from build123d import *

# Parameters (mm, degrees)
SKETCH2_W           = 154.686
SKETCH2_H           = 228.6
BOSS_EXTRUDE1_DEPTH = 6.35
SKETCH1_R           = 2.2225
CUT_EXTRUDE1_DEPTH  = 6.35
SKETCH3_W           = 15.24
SKETCH3_H           = 50.8
CUT_EXTRUDE2_DEPTH  = 6.35
SKETCH8_R           = 2.54
CUT_EXTRUDE3_DEPTH  = 17.78
SKETCH9_R           = 1.5875
CUT_EXTRUDE4_DEPTH  = 17.78
SKETCH10_R          = 1.5875
CUT_EXTRUDE5_DEPTH  = 10.16
SKETCH12_W          = 3.048
SKETCH12_H          = 18.542
CUT_EXTRUDE7_DEPTH  = 8.255


with BuildPart() as part:
    # Sketch2 → Boss-Extrude1 (new body)
    with BuildSketch(Plane(origin=(0, 0, 0), x_dir=(1, 0, 0), z_dir=(0, 1, 0))):
        with Locations((26.543, 26.944051327)):
            Rectangle(SKETCH2_W, SKETCH2_H)
    extrude(amount=BOSS_EXTRUDE1_DEPTH)

    # Sketch1 → Cut-Extrude1 (cut)
    with BuildSketch(Plane(origin=(0, 0, 0), x_dir=(1, 0, 0), z_dir=(0, 1, 0))):
        with Locations((0, 90.444051327)):
            Circle(SKETCH1_R)
        with Locations((53.086, 90.444051327)):
            Circle(SKETCH1_R)
        Circle(SKETCH1_R)
        with Locations((53.086, 0)):
            Circle(SKETCH1_R)
    extrude(amount=CUT_EXTRUDE1_DEPTH, mode=Mode.SUBTRACT)

    # Sketch3 → Cut-Extrude2 (cut)
    with BuildSketch(Plane(origin=(0, 6.35, 0), x_dir=(1, 0, 0), z_dir=(0, 1, 0))):
        with Locations((96.266, 56.154051327)):
            Rectangle(SKETCH3_W, SKETCH3_H)
        with Locations((-43.18, 56.154051327)):
            Rectangle(SKETCH3_W, SKETCH3_H)
    extrude(amount=-CUT_EXTRUDE2_DEPTH, mode=Mode.SUBTRACT)

    # Sketch8 → Cut-Extrude3 (cut)
    with BuildSketch(Plane(origin=(0, 6.35, 0), x_dir=(1, 0, 0), z_dir=(0, 1, 0))):
        with Locations((26.550112, -20.29968)):
            Circle(SKETCH8_R)
        with Locations((-23.077082804, 0.02032)):
            Circle(SKETCH8_R)
        with Locations((76.177306804, 0.02032)):
            Circle(SKETCH8_R)
    extrude(amount=-CUT_EXTRUDE3_DEPTH, mode=Mode.SUBTRACT)

    # Sketch9 → Cut-Extrude4 (cut)
    with BuildSketch(Plane(origin=(0, 6.35, 0), x_dir=(1, 0, 0), z_dir=(0, 1, 0))):
        with Locations((53.722112, -33.005948673)):
            Circle(SKETCH9_R)
        with Locations((5.722112, -33.005948673)):
            Circle(SKETCH9_R)
        with Locations((53.722112, -81.005948673)):
            Circle(SKETCH9_R)
        with Locations((5.722112, -81.005948673)):
            Circle(SKETCH9_R)
    extrude(amount=-CUT_EXTRUDE4_DEPTH, mode=Mode.SUBTRACT)

    # Sketch10 → Cut-Extrude5 (cut)
    with BuildSketch(Plane(origin=(0, 6.35, 0), x_dir=(1, 0, 0), z_dir=(0, 1, 0))):
        with Locations((-22.3266, 105.430051327)):
            Circle(SKETCH10_R)
        with Locations((-22.3266, -21.569948673)):
            Circle(SKETCH10_R)
        with Locations((75.4126, 105.430051327)):
            Circle(SKETCH10_R)
        with Locations((75.4126, -21.569948673)):
            Circle(SKETCH10_R)
    extrude(amount=-CUT_EXTRUDE5_DEPTH, mode=Mode.SUBTRACT)

    # Sketch12 → Cut-Extrude7 (cut)
    with BuildSketch(Plane(origin=(0, 6.35, 0), x_dir=(1, 0, 0), z_dir=(0, 1, 0))):
        with Locations((-0.373888, 19.451051327)):
            Rectangle(SKETCH12_W, SKETCH12_H)
        with Locations((-0.373888, 70.759051327)):
            Rectangle(SKETCH12_W, SKETCH12_H)
        with Locations((53.474112, 71.267051327)):
            Rectangle(SKETCH12_W, SKETCH12_H)
        with Locations((53.474112, 18.943051327)):
            Rectangle(SKETCH12_W, SKETCH12_H)
    extrude(amount=-CUT_EXTRUDE7_DEPTH, mode=Mode.SUBTRACT)


solid = part.part
Verification items for the finished model (mm, model axes). A direction names the side the tool comes from. Give positions to 0.01 mm unless a question says otherwise; leave off trailing zeros. Order: outer loops, then holes, each group sorted by start corner. A loop starts at its lowest first (then second) coordinate and runs counter-clockwise, first axis right, second up. Notation, with made-up numbers: M -40,88 L -36,88 A30 ccw -36,119 Z; hole C 38.25,77.5 d3. An arc over 180 degrees is marked long. Use one line per item in the form item = value. Start each with the question number.
Q1. Section check A-A (z = -14.5). Enter the section's corners in (x, y).
Q2. Access from +Z, -Z, +X, -X, +Y, -Y to the whole of each face (thin tool, end or side, straight path). Record for faces 1 (the flat face through (51.95, 3, -71)), 2 (the flat face through (88.646, 3, -56)), 3 (the flat face through (-43, 3, -81.554)), 4 (the flat face through (103.886, 3, 29)), 5 (the flat face through (25, 0, -29)).
Q3. Scan lines: line 1 along Z through (x, y) = (0, 4); line 2 along X through (y, z) = (1.5, 0); line 3 along X through (y, z) = (4, -74.5). Record each from-to range of solid material in increasing order. Write a range as [from, to].
Q4. Mould release check, pull along X, two halves, no side actions. Record for faces 6 (the cylindrical face through (50.866, 3.131, -0.098)), 7 (the flat face through (51.95, 3, -19)), 8 (the flat face through (96, 3, -30.754)), 9 (the flat face through (-35.56, 3, -56)): +X half, -X half, draft (parallel to the pull), parting line (faces both ways), or undercut.
Q5. Section check B-B (y = 1.25). Count the separate pieces of the cut face and the enclosed holes in it, then the cut area to 3 significant figures.
Q6. Go/stop test with flat-tipped pins: pin 1 Ø10 at (x, z) = (-15.5, -71) entering from -Y; pin 2 Ø3 at (y, z) = (1.5, -36) entering from -X; pin 3 Ø3 at (y, z) = (3.5, -64.5) entering from +X. Record where each tip stops, or that it passes through.
Evaluation:
q1.outline = M -50.8,0 L -1.9,0 L -1.9,6.35 L -50.8,6.35 Z; M 1.15,0 L 51.95,0 L 51.95,6.35 L 1.15,6.35 Z; M 55,0 L 103.89,0 L 103.89,6.35 L 55,6.35 Z
q2.face_1 = +Y, -Y
q2.face_2 = +X, +Y, -Y
q2.face_3 = -X, +Y, -Y
q2.face_4 = +Z, -Z, +X, +Y, -Y
q2.face_5 = +Z, -Z, +X, -X, -Y
q3.line_1 = [-141.24, -92.67], [-88.22, -80.03], [-61.49, -28.72], [-10.18, -2.22], [2.22, 87.36]
q3.line_2 = [-50.8, -25.62], [-20.54, -2.22], [2.22, 50.86], [55.31, 73.64], [78.72, 103.89]
q3.line_3 = [-35.56, -1.9], [1.15, 51.95], [55, 88.65]
q4.face_6 = undercut
q4.face_7 = undercut
q4.face_8 = draft
q4.face_9 = -X half
q5.separate_pieces = 1
q5.enclosed_holes = 19
q5.area = 33,400 mm2
q6.pin_1 = 0
q6.pin_2 = -35.56
q6.pin_3 = 88.65
